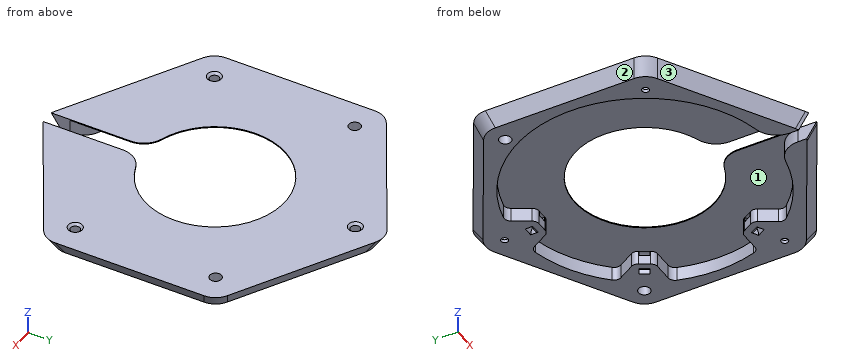
from build123d import *

# Parameters (mm, degrees)
BOSS_EXTRUDE1_DEPTH       = 6.4
BOSS_EXTRUDE1_DRAFT       = -30
FILLET1_R                 = 10
SKETCH13_R                = 2
CUT_EXTRUDE3_DEPTH        = 5
SKETCH14_R                = 1.5
CUT_EXTRUDE4_DEPTH        = 97.51813456
SKETCH15_R                = 55
CUT_EXTRUDE5_DEPTH        = 6
CIRPATTERN9_COUNT         = 3
BOSS_EXTRUDE4_DEPTH       = 6
SKETCH21_W                = 4
SKETCH21_H                = 2
FILLET8_R                 = 1
CIRPATTERN11_COUNT        = 3
CIRPATTERN11_ANGLE        = 120
FILLET8_OF_CIRPATTERN11_R = 1
SKETCH16_R                = 2.5
CUT_EXTRUDE6_DEPTH        = 97.51813456
CIRPATTERN10_COUNT        = 3
CUT_EXTRUDE7_DEPTH        = 97.51813456
FILLET9_R                 = 10
FILLET10_R                = 3
CHAMFER2_SIZE             = 1


with BuildPart() as part:
    # Sketch1 → Boss-Extrude1 (with draft: the straight prism first)
    with BuildSketch(Plane.XY):
        Polygon((0, 69.282032303), (-60, 34.641016151), (-60, -34.641016151), (0, -69.282032303), (60, -34.641016151), (60, 34.641016151), align=None)
    extrude(amount=BOSS_EXTRUDE1_DEPTH)
    # Boss-Extrude1: the draft: its side faces are tilted about the plane it starts from
    boss_extrude1_sides = [part.faces().sort_by_distance(p)[0] for p in [
        (-30, 51.961524227, 3.2),
        (-60, 0, 3.2),
        (-30, -51.961524227, 3.2),
        (30, -51.961524227, 3.2),
        (60, 0, 3.2),
        (30, 51.961524227, 3.2),
    ]]
    draft(boss_extrude1_sides, Plane.XY, BOSS_EXTRUDE1_DRAFT)

    # Fillet1
    fillet1_edges = [part.edges().sort_by_distance(p)[0] for p in [
        (61.847520861, 35.707682818, 3.2),
        (61.847520861, -35.707682818, 3.2),
        (0, -71.415365636, 3.2),
        (-61.847520861, -35.707682818, 3.2),
        (-61.847520861, 35.707682818, 3.2),
        (0, 71.415365636, 3.2),
    ]]
    fillet(fillet1_edges, radius=FILLET1_R)

    # Sketch13 → Cut-Extrude3 (cut)
    with BuildSketch(Plane.XY.offset(6.4)):
        with Locations((0, 60)):
            Circle(SKETCH13_R)
    cut_extrude3 = extrude(amount=-CUT_EXTRUDE3_DEPTH, mode=Mode.SUBTRACT)

    # Sketch14 → Cut-Extrude4 (cut, through all)
    with BuildSketch(Plane(origin=(0, 0, 0), x_dir=(-1, 0, 0), z_dir=(0, 0, -1))):
        with Locations((0, 60)):
            Circle(SKETCH14_R)
    cut_extrude4 = extrude(amount=-CUT_EXTRUDE4_DEPTH, mode=Mode.SUBTRACT)

    # Sketch15 → Cut-Extrude5 (cut)
    with BuildSketch(Plane(origin=(0, 0, 0), x_dir=(-1, 0, 0), z_dir=(0, 0, -1))):
        Circle(SKETCH15_R)
    extrude(amount=-CUT_EXTRUDE5_DEPTH, mode=Mode.SUBTRACT)

    # CirPattern9: Cut-Extrude3, Cut-Extrude4 ×3 about axis
    cirpattern9_axis = Axis((0, 0, 0), (0, 0, 1))
    add([cut_extrude3.rotate(cirpattern9_axis, i * 360 / CIRPATTERN9_COUNT) for i in range(1, CIRPATTERN9_COUNT)], mode=Mode.SUBTRACT)
    add([cut_extrude4.rotate(cirpattern9_axis, i * 360 / CIRPATTERN9_COUNT) for i in range(1, CIRPATTERN9_COUNT)], mode=Mode.SUBTRACT)

    # Sketch20 → Boss-Extrude4 (add)
    with BuildSketch(Plane(origin=(0, 0, 6), x_dir=(-1, 0, 0), z_dir=(0, 0, -1))):
        Polygon((-12.082903769, 58), (-4, 44), (4, 44), (12.082903769, 58), align=None)
    boss_extrude4 = extrude(amount=BOSS_EXTRUDE4_DEPTH)

    # Sketch21 → Cut-Revolve1 (revolve, cut)
    with BuildSketch(Plane(origin=(0, 44, 0), x_dir=(-1, 0, 0), z_dir=(0, -1, 0))):
        with Locations((0, -5)):
            Rectangle(SKETCH21_W, SKETCH21_H)
    cut_revolve1 = revolve(axis=Axis((4, 44, 0), (1, 0, 0)), mode=Mode.SUBTRACT)

    # Fillet8
    fillet8_edges = [part.edges().sort_by_distance(p)[0] for p in [
        (0, 48, 0),
    ]]
    fillet(fillet8_edges, radius=FILLET8_R)

    # CirPattern11: Boss-Extrude4, Cut-Revolve1 ×3 about axis
    cirpattern11_axis = Axis((0, 0, 0), (0, 0, -1))
    add([boss_extrude4.rotate(cirpattern11_axis, i * CIRPATTERN11_ANGLE / (CIRPATTERN11_COUNT - 1)) for i in range(1, CIRPATTERN11_COUNT)])
    add([cut_revolve1.rotate(cirpattern11_axis, i * CIRPATTERN11_ANGLE / (CIRPATTERN11_COUNT - 1)) for i in range(1, CIRPATTERN11_COUNT)], mode=Mode.SUBTRACT)

    # Fillet8 of CirPattern11
    fillet8_of_cirpattern11_edges = [part.edges().sort_by_distance(p)[0] for p in [
        (41.569219382, 24, 0),
        (41.569219382, -24, 0),
    ]]
    fillet(fillet8_of_cirpattern11_edges, radius=FILLET8_OF_CIRPATTERN11_R)

    # Sketch16 → Cut-Extrude6 (cut, through all)
    with BuildSketch(Plane(origin=(0, 0, 0), x_dir=(-1, 0, 0), z_dir=(0, 0, -1))):
        with Locations((0, -60)):
            Circle(SKETCH16_R)
    cut_extrude6 = extrude(amount=-CUT_EXTRUDE6_DEPTH, mode=Mode.SUBTRACT)

    # CirPattern10: Cut-Extrude6 ×3 about axis
    cirpattern10_axis = Axis((0, 0, 0), (0, 0, 1))
    for i in range(1, CIRPATTERN10_COUNT):
        add(cut_extrude6.rotate(cirpattern10_axis, i * 360 / CIRPATTERN10_COUNT), mode=Mode.SUBTRACT)

    # Sketch22 → Cut-Extrude7 (cut, through all)
    with BuildSketch(Plane.XY.offset(6.4)):
        with BuildLine():
            Line((-3, -37.828560639), (-3, -80))
            Line((-3, -80), (3, -80))
            Line((3, -80), (3, -37.828560639))
            ThreePointArc((3, -37.828560639), (4.860589702, -32.019085619), (9.75, -28.371420479))
            ThreePointArc((9.75, -28.371420479), (0, 30), (-9.75, -28.371420479))
            ThreePointArc((-9.75, -28.371420479), (-4.860589702, -32.019085619), (-3, -37.828560639))
        make_face()
    extrude(amount=-CUT_EXTRUDE7_DEPTH, mode=Mode.SUBTRACT)

    # Fillet9
    fillet9_edges = [part.edges().sort_by_distance(p)[0] for p in [
        (3, -54.918120871, 3),
        (-3, -54.918120871, 3),
    ]]
    fillet(fillet9_edges, radius=FILLET9_R)

    # Fillet10
    fillet10_edges = [part.edges().sort_by_distance(p)[0] for p in [
        (51.782434001, 18.535898385, 3),
        (41.943775884, 35.576954122, 3),
        (36.105117767, 25.464101615, 3),
        (40.105117767, 18.535898385, 3),
        (41.943775884, -35.576954122, 3),
        (51.782434001, -18.535898385, 3),
        (40.105117767, -18.535898385, 3),
        (36.105117767, -25.464101615, 3),
        (9.838658117, 54.112852507, 3),
        (-9.838658117, 54.112852507, 3),
        (-4, 44, 3),
        (4, 44, 3),
    ]]
    fillet(fillet10_edges, radius=FILLET10_R)

    # Chamfer2
    # the kernel refuses this chamfer: 1 mm, written as the material it takes off along each edge
    with BuildSketch(Plane(origin=(0, 60, 6.4), x_dir=(1, 0, 0), z_dir=(0, -1, 0))) as chamfer2_piece_1:
        Polygon((2 + CHAMFER2_SIZE, 0), (2, -CHAMFER2_SIZE), (2, 0), align=None)
    revolve(axis=Axis((0, 60, 6.4), (0, 0, 1)), mode=Mode.SUBTRACT)
    with BuildSketch(Plane(origin=(51.961524227, -30, 6.4), x_dir=(-0.4999999999999998, -0.8660254037844389, 0), z_dir=(-0.8660254037844389, 0.4999999999999998, 0))) as chamfer2_piece_2:
        Polygon((2 + CHAMFER2_SIZE, 0), (2, -CHAMFER2_SIZE), (2, 0), align=None)
    revolve(axis=Axis((51.961524227, -30, 6.4), (0, 0, 1)), mode=Mode.SUBTRACT)
    with BuildSketch(Plane(origin=(-51.961524227, -30, 6.4), x_dir=(-0.4999999999999998, 0.8660254037844389, 0), z_dir=(0.8660254037844389, 0.4999999999999998, 0))) as chamfer2_piece_3:
        Polygon((2 + CHAMFER2_SIZE, 0), (2, -CHAMFER2_SIZE), (2, 0), align=None)
    revolve(axis=Axis((-51.961524227, -30, 6.4), (0, 0, 1)), mode=Mode.SUBTRACT)


solid = part.part
The listing builds one solid part. Answer for the finished solid, in the listing's coordinates (mm). Face numbers are marked on the shaded views. Give positions to 0.01 mm unless a question says otherwise; leave off trailing zeros. Write each loop counter-clockwise with the first axis right and the second up, starting at its lowest first coordinate (ties: lowest second). Pieces come first, ordered by that corner, then holes. Notation, with made-up numbers: (78, -16.5) - (111, -16.5) arc R18 cw to (111, 9.5) - close; hole circle Ø9 at (53.25, 29.5). An arc over 180 degrees is marked (long way). One line per question, with ' | ' between items. Start each with the question number.
1. Section D-D, the plane z = 3 is taken. Count the separate pieces of the cut face and the enclosed holes in it, then the cut area to 3 significant figures.
2. Section A-A, the plane y = 0 is taken. Determine the outline of the cut face in (x, z), then the cut area to 3 significant figures.
3. Section C-C, the plane x = 46.5 is taken. Determine the outline of the cut face in (y, z).
4. Given P1, Ø1.5, axis at y = 18, z = 0.5, coming from the +X side; P2, Ø8, axis at x = 16.5, y = 33.5, coming from the -Z side; P3, Ø3.5, axis at x = 51.96, y = -30, coming from the +Z side, each flat-ended and moving along its own axis, determine where each tip first touches the part or whether it passes through.
5. Determine the mould class of the marked faces 1, 2 and 3 for opening direction Y: +Y half, -Y half, draft (parallel to the pull), parting line (faces both ways), or undercut.
6. Section B-B, the plane x = 23 is taken. Determine the outline of the cut face in (y, z), then the cut area to 3 significant figures.
7. Straight lines are drawn through the part: line 1 (Y direction, x = 43, z = 3.75); line 2 (Y direction, x = 0, z = 3.6); line 3 (X direction, y = -30, z = 3.1). For each, find the intervals that lie inside material, in ascending order.
Result:
1) separate pieces: 1 | enclosed holes: 8 | area: 3,910 mm2
2) outline: (-63.7, 6.4) - (-60, 0) - (-55, 0) - (-55, 6) - (-30, 6) - (-30, 6.4) - close; (30, 6) - (55, 6) - (55, 0) - (60, 0) - (63.7, 6.4) - (30, 6.4) - close | area: 108 mm2
3) outline: (-46.7, 6.4) - (-42.44, 0) - (-18.54, 0) - (-18.54, 6) - (18.54, 6) - (18.54, 0) - (42.44, 0) - (46.7, 6.4) - close
4) P1: stops at x = 60.72 | P2: stops at z = 6 | P3: stops at z = 1.4
5) face 1: undercut | face 2: draft | face 3: -Y half
6) outline: (-60.27, 6.4) - (-56, 0) - (-49.96, 0) - (-49.96, 6) - (-19.26, 6) - (-19.26, 6.4) - close; (19.26, 6) - (49.96, 6) - (49.96, 0) - (56, 0) - (60.27, 6.4) - (19.26, 6.4) - close | area: 129 mm2
7) line 1: y = -46.96 to -22.89, -22.52 to -18.54, 18.54 to 22.52, 22.89 to 46.96 | line 2: y = 44 to 45.74, 48.8 to 58, 62 to 70.37 | line 3: x = -61.79 to -53.96, -49.96 to -46.1, 38.72 to 49.96, 53.96 to 61.79
